```python
from build123d import *

# Parameters (mm, degrees)
F0_W     = 31.75
F0_H     = 127
F1_DEPTH = 31.75
F2_W     = 8.89
F2_H     = 57.15
F3_DEPTH = 10.16
F5_DEPTH = 10.16


with BuildPart() as f1:
    # F0 (on Top) → F1 (new body)
    with BuildSketch(Plane.XY):
        with Locations((15.875, 63.5)):
            Rectangle(F0_W, F0_H)
    extrude(amount=F1_DEPTH)

    # F2 (on face) → F3 (cut)
    with BuildSketch(Plane.XY.offset(31.75)):
        with Locations((15.875, 34.925)):
            Rectangle(F2_W, F2_H)
    extrude(amount=-F3_DEPTH, mode=Mode.SUBTRACT)

    # F4 (on face) → F5 (cut, through all)
    with BuildSketch(Plane.XY.offset(31.75)):
        with BuildLine():
            ThreePointArc((15.875, 58.966207), (19.339109, 58.263056), (21.306743, 61.199532))
            ThreePointArc((21.306743, 61.199532), (19.339109, 64.136008), (15.875, 63.432856))
            ThreePointArc((15.875, 63.432856), (16.554733, 62.406898), (16.793257, 61.199532))
            ThreePointArc((16.793257, 61.199532), (16.554733, 59.992165), (15.875, 58.966207))
        make_face()
        with BuildLine():
            ThreePointArc((15.875, 58.966207), (14.956743, 61.199532), (15.875, 63.432856))
            ThreePointArc((15.875, 63.432856), (10.443257, 61.199532), (15.875, 58.966207))
        make_face()
        with BuildLine():
            ThreePointArc((15.875, 6.417144), (19.339109, 5.713992), (21.306743, 8.650468))
            ThreePointArc((21.306743, 8.650468), (19.339109, 11.586944), (15.875, 10.883793))
            ThreePointArc((15.875, 10.883793), (16.554733, 9.857835), (16.793257, 8.650468))
            ThreePointArc((16.793257, 8.650468), (16.554733, 7.443102), (15.875, 6.417144))
        make_face()
        with BuildLine():
            ThreePointArc((15.875, 6.417144), (14.956743, 8.650468), (15.875, 10.883793))
            ThreePointArc((15.875, 10.883793), (10.443257, 8.650468), (15.875, 6.417144))
        make_face()
    extrude(amount=-F5_DEPTH, mode=Mode.SUBTRACT)


solid = f1.part
```
Work out the finished part from the listing and answer in its coordinate system (mm). A direction names the side the tool comes from. Round coordinates to 2 decimals unless told otherwise and drop trailing zeros. Write each loop counter-clockwise with the first axis right and the second up, starting at its lowest first coordinate (ties: lowest second). Pieces come first, ordered by that corner, then holes. Notation, with made-up numbers: (-36, -24) -> (-29, -24) arc R22 ccw to (-29, -11) -> close; hole circle Ø7 at (89, 60). An arc over 180 degrees is marked (long way). Write each question's results on one line, items separated by ' | '.
1) The part is cut by section A-A (z = 30). Write down the section's boundary in (x, y) (3 decimals).
Findings:
outline: (0, 0) -> (31.75, 0) -> (31.75, 127) -> (0, 127) -> close; hole (11.43, 10.951) arc R3.175 ccw to (15.807, 6.35) -> (15.943, 6.35) arc R3.175 ccw to (20.32, 10.951) -> (20.32, 58.899) arc R3.175 ccw to (15.943, 63.5) -> (15.807, 63.5) arc R3.175 ccw to (11.43, 58.899) -> close
2) The part is cut by section B-B (y = 46). Write down the section's boundary in (x, z).
Findings:
outline: (0, 0) -> (31.75, 0) -> (31.75, 31.75) -> (20.32, 31.75) -> (20.32, 21.59) -> (11.43, 21.59) -> (11.43, 31.75) -> (0, 31.75) -> close
3) For a pull along X with two mould halves and no side action, classify faces 3 (the flat face through (16, 35, 21.59)), 4 (the flat face through (0, 63, 16)), 5 (the flat face through (31.75, 63, 16)) as +X half, -X half, draft (parallel to the pull), parting line (faces both ways), or undercut.
Findings:
face 3: undercut | face 4: -X half | face 5: +X half
4) A flat-ended cylindrical pin translates along its axis: pin 1 (3.5 mm diameter, centred on x = 18.5, y = 47.5, fed in from +Z). Find the tip coordinate at first contact, or state that the pin passes through.
Findings:
pin 1: stops at z = 21.59
5) Which of the six approach directions +Z, -Z, +X, -X, +Y, -Y give full straight-line access (tool end or side, diameter ignored) to faces 1 (the flat face through (20.32, 35, 27)), 2 (the flat face through (16, 127, 16))?
Findings:
face 1: +Z | face 2: +Z, -Z, +X, -X, +Y
6) Consider line 1 along X through (y, z) = (24, 29.5); line 2 along Y through (x, z) = (19.5, 28.5); line 3 along X through (y, z) = (6.5, 27). Determine where each line is inside the solid, lowest interval first. Write a range as [from, to].
Findings:
line 1: x = [0, 11.43], [20.32, 31.75] | line 2: y = [0, 5.79], [64.06, 127] | line 3: x = [0, 11.28], [20.47, 31.75]
